Check sheet for the modelled part. Datum: model origin and axes. Units: mm. Round coordinates to 2 decimals unless told otherwise and drop trailing zeros. Write each loop counter-clockwise with the first axis right and the second up, starting at its lowest first coordinate (ties: lowest second). Pieces come first, ordered by that corner, then holes. Notation, with made-up numbers: (12.25, 38) -> (52.25, 38) arc R9 cw to (52.25, 51) -> close; hole circle Ø9 at (12, 67). An arc over 180 degrees is marked (long way). Answer as a JSON object with one key per item and string values. Group by question number.
```python
from build123d import *

# Parameters (mm, degrees)
CIRCLE002_AS_DRAWN_R                         = 2.5
EXTRUDE004_DEPTH                             = 10
EXTRUDE004_ONTO_CIRCLE002_ROLL_ANGLE         = 135.690278
EXTRUDE004_ONTO_CIRCLE002_PITCH_ANGLE        = 0
EXTRUDE004_ONTO_CIRCLE002_PLACEMENT_ANGLE    = 90.000001
CIRCLE001_AS_DRAWN_R                         = 2.5
EXTRUDE003_DEPTH                             = 10
EXTRUDE003_ONTO_CIRCLE001_ROLL_ANGLE         = 135.690278
EXTRUDE003_ONTO_CIRCLE001_PITCH_ANGLE        = 0
EXTRUDE003_ONTO_CIRCLE001_PLACEMENT_ANGLE    = 90.000001
RECTANGLE001_AS_DRAWN_W                      = 150
RECTANGLE001_AS_DRAWN_H                      = 6
EXTRUDE002_DEPTH                             = 20
EXTRUDE002_ONTO_RECTANGLE001_ROLL_ANGLE      = 89.999995
EXTRUDE002_ONTO_RECTANGLE001_PITCH_ANGLE     = -44.309723
EXTRUDE002_ONTO_RECTANGLE001_PLACEMENT_ANGLE = 3e-06


with BuildPart() as extrude004:
    # Circle002 as drawn → Extrude004 (new)
    with BuildSketch(Plane.XY):
        Circle(CIRCLE002_AS_DRAWN_R)
    extrude(amount=-EXTRUDE004_DEPTH)


with BuildPart() as extrude004_1:
    # Extrude004 onto Circle002 roll: moved
    add(extrude004.part.rotate(Axis((0, 0, 0), (1, 0, 0)), EXTRUDE004_ONTO_CIRCLE002_ROLL_ANGLE))


with BuildPart() as extrude004_2:
    # Extrude004 onto Circle002 pitch: moved
    add(extrude004_1.part.rotate(Axis((0, 0, 0), (0, 1, 0)), EXTRUDE004_ONTO_CIRCLE002_PITCH_ANGLE))


with BuildPart() as extrude004_3:
    # Extrude004 onto Circle002 placement: moved
    add(extrude004_2.part.moved(Location((53.611526, -9.999937, 1187.461103))).rotate(Axis((53.611526, -9.999937, 1187.461103), (0, 0, 1)), EXTRUDE004_ONTO_CIRCLE002_PLACEMENT_ANGLE))


with BuildPart() as compound001:
    # Circle001 as drawn → Extrude003 (new)
    with BuildSketch(Plane.XY):
        Circle(CIRCLE001_AS_DRAWN_R)
    extrude(amount=-EXTRUDE003_DEPTH)


with BuildPart() as compound001_1:
    # Extrude003 onto Circle001 roll: moved
    add(compound001.part.rotate(Axis((0, 0, 0), (1, 0, 0)), EXTRUDE003_ONTO_CIRCLE001_ROLL_ANGLE))


with BuildPart() as compound001_2:
    # Extrude003 onto Circle001 pitch: moved
    add(compound001_1.part.rotate(Axis((0, 0, 0), (0, 1, 0)), EXTRUDE003_ONTO_CIRCLE001_PITCH_ANGLE))


with BuildPart() as compound001_3:
    # Extrude003 onto Circle001 placement: moved
    add(compound001_2.part.moved(Location((125.168938, -9.99992, 1257.314767))).rotate(Axis((125.168938, -9.99992, 1257.314767), (0, 0, 1)), EXTRUDE003_ONTO_CIRCLE001_PLACEMENT_ANGLE))

    # Compound001: union Extrude004
    add(extrude004_3.part)


with BuildPart() as compound001_4:
    # Compound001 placement: moved
    add(compound001_3.part.moved(Location((0, -401.000072, 0))))


with BuildPart() as cut001:
    # Rectangle001 as drawn → Extrude002 (new, symmetric)
    with BuildSketch(Plane.XY):
        with Locations((75, 3)):
            Rectangle(RECTANGLE001_AS_DRAWN_W, RECTANGLE001_AS_DRAWN_H)
    extrude(amount=EXTRUDE002_DEPTH, both=True)


with BuildPart() as cut001_1:
    # Extrude002 onto Rectangle001 roll: moved
    add(cut001.part.rotate(Axis((0, 0, 0), (1, 0, 0)), EXTRUDE002_ONTO_RECTANGLE001_ROLL_ANGLE))


with BuildPart() as cut001_2:
    # Extrude002 onto Rectangle001 pitch: moved
    add(cut001_1.part.rotate(Axis((0, 0, 0), (0, 1, 0)), EXTRUDE002_ONTO_RECTANGLE001_PITCH_ANGLE))


with BuildPart() as cut001_3:
    # Extrude002 onto Rectangle001 placement: moved
    add(cut001_2.part.moved(Location((35.72217, -9.99993, 1169.997685))).rotate(Axis((35.72217, -9.99993, 1169.997685), (0, 0, 1)), EXTRUDE002_ONTO_RECTANGLE001_PLACEMENT_ANGLE))


with BuildPart() as cut001_4:
    # Extrude002 placement: moved
    add(cut001_3.part.moved(Location((0, -401.000072, 0))))

    # Cut001: cut Compound001
    add(compound001_4.part, mode=Mode.SUBTRACT)


solid = cut001_4.part
```
(1) Section check A-A on x = 100. Record the cut outline in (y, z), then the cut area to 3 significant figures.
(2) Section check B-B on y = -424.5. Record the cut outline in (x, z), then the cut area to 3 significant figures.
(3) Release check for a two-part mould opening along Y. For faces 1 (the flat face through (140.992, -411.28, 1276.895)), 2 (the flat face through (87, -431, 1224)), 3 (the cylindrical face through (121.356, -411.542, 1257.727)) record: pulls with the +Y half, pulls with the -Y half, needs draft (parallel to the pull), parting line crosses it, or undercut.
(4) Go/stop test with flat-tipped pins: pin 1 Ø5 at (y, z) = (-423, 1262) entering from -X; pin 2 Ø4 at (x, y) = (88.5, -426.5) entering from +Z; pin 3 Ø3 at (y, z) = (-415.5, 1209) entering from -X. Record where each tip stops, or that it passes through.
(5) Scan lines: line 1 along Z through (x, y) = (95.5, -429); line 2 along Z through (x, y) = (70.5, -412); line 3 along X through (y, z) = (-429, 1192). Record each from-to range of solid material in increasing order.
Data:
{
 "1": {"outline": "(-431, 1232.75) -> (-391, 1232.75) -> (-391, 1241.13) -> (-431, 1241.13) -> close", "area": "335 mm²"},
 "2": {"outline": "(31.53, 1174.29) -> (35.72, 1170) -> (143.06, 1274.78) -> (138.87, 1279.07) -> close", "area": "900 mm²"},
 "3": {"face 1": "needs draft", "face 2": "pulls with the -Y half", "face 3": "undercut"},
 "4": {"pin 1": "stops at x = 118.82", "pin 2": "stops at z = 1231.86", "pin 3": "stops at x = 65.55"},
 "5": {"line 1": "z = 1228.35 to 1236.74", "line 2": "z = 1203.95 to 1212.33", "line 3": "x = 49.67 to 58.26"}
}
